Part model, mm, in its own coordinate system. A direction names the side the tool comes from. Give positions to 0.01 mm unless a question says otherwise; leave off trailing zeros. Write each loop counter-clockwise with the first axis right and the second up, starting at its lowest first coordinate (ties: lowest second). Pieces come first, ordered by that corner, then holes. Notation, with made-up numbers: M -33.5,-13.75 L -12.5,-13.75 A21 ccw -12.5,-4.75 Z; hole C 44,83.25 d2. An arc over 180 degrees is marked long. Answer as CSV lines item,"result". Start each with the question number.
1) Slice it at A-A, the plane z = 24. Give the cut face in (x, y), plus the area to 3 significant figures.
2) Tool access for faces 5 (the cylindrical face through (-3.22, -24.54, 1.43)), 6 (the cylindrical face through (0, -2, 58)): list every direction of +Z, -Z, +X, -X, +Y, -Y with a clear straight run to the whole face (end or side of a thin tool).
3) Mould opens along X. For faces 1 (the cylindrical face through (-4.336, 19.524, 1.43)), 2 (the flat face through (-1.9, -20.1, 0)), 3 (the conical face through (-2.579, -19.641, 37.395)), 4 (the flat face through (0, 0, 2.9)) say: pulls with the +X half, pulls with the -X half, needs draft (parallel to the pull), parting line crosses it, or undercut.
4) Pin check, flat tips, straight feed: pin 1 Ø3 at (y, z) = (-4.5, 25) entering from +X; pin 2 Ø8 at (y, z) = (16.5, 36.5) entering from -X; pin 3 Ø1.5 at (y, z) = (-10, 34.5) entering from -X; pin 4 Ø6 at (x, z) = (8, 53.5) entering from -Y. Stop position of each tip, or through.
5) Wall check: line 1 along Y through (x, z) = (0, 1.7); line 2 along Z through (x, y) = (3.5, -9.5); line 3 along Z through (x, y) = (16, -18.5). Give the ranges that are in metal, low to high. Write a range as from..to.
Autodesk Fusion 360 part; units mm, degrees
sketch "Skizze1" plane through (0, 0, 0) normal (0, 0, 1) x (1, 0, 0)
  circle A0 centre (0, 0) radius 24.75
  circle A1 centre (0, 0) radius 20
  dimension "d1" = 49.5
  dimension "d4" = 40
extrude "Extrusion1" add sketch "Skizze1" along normal blind 2.9
sketch "Skizze2" plane through (0, 0, 0) normal (0, 1, 0) x (1, 0, 0)
  line L0 (-24.75, -2.9) -> (24.75, -2.9)
  line L1 (-24.75, 0) -> (24.75, 0)
  line L2 (22.65, -2.9) -> (22.65, -7.9)
  line L3 (22.65, -7.9) -> (22.65, -12.9)
  line L4 (22.65, -12.9) -> (22.65, -17.9)
  line L5 (22.65, -17.9) -> (22.5, -22.8977)
  line L6 (22.5, -22.8977) -> (22, -27.8727)
  line L7 (22, -27.8727) -> (21.15, -32.7999)
  line L8 (21.15, -32.7999) -> (19.75, -37.5999)
  line L9 (19.75, -37.5999) -> (18.1, -42.3198)
  line L10 (0, -2.9) -> (0, -41.75) construction
  line L11 (18.1, -42.3198) -> (15.05, -49.9)
  line L12 (15.05, -49.9) -> (0, -49.9)
  line L13 (0, -49.9) -> (0, -2.9)
  dimension "d6" = 5
  dimension "d8" = 22.65
  dimension "d9" = 22.65
  dimension "d10" = 22.65
  dimension "d11" = 22.65
  dimension "d12" = 22.5
  dimension "d13" = 22
  dimension "d14" = 21.15
  dimension "d15" = 19.75
  dimension "d17" = 18.1
  dimension "d18" = 47
  dimension "d20" = 15.05
  dimension "d21" = 8.1708
  dimension "d22" = 7.5802
revolve "Drehen1" add sketch "Skizze2" angle 360 about axis through (0, 0, 49.9) along (0, 0, -1)
fillet "Abrundung1" radius 28 6 edges at (-16.8751, -6.5452, 42.3198) (-18.4135, -7.1419, 37.5999) (-19.7187, -7.6482, 32.7999) (-20.5112, -7.9555, 27.8727) (-20.9774, -8.1363, 22.8977) (-21.1172, -8.1906, 17.9)
fillet "Abrundung2" radius 1 1 edges at (-21.1172, 8.1906, 2.9)
sketch "Skizze3" plane through (0, 0, 49.9) normal (0, 0, 1) x (-1, 0, 0)
  circle A0 centre (0, 0) radius 15.05
  circle A1 centre (0, 0) radius 2
  dimension "d28" = 4
extrude "Extrusion2" add sketch "Skizze3" along normal blind 16 contours A1
equation "d8 = ( 45.3 / 2 ) * 1 mm"
equation "d9 = ( 45.3 / 2 ) * 1 mm"
equation "d10 = ( 45.3 / 2 ) * 1 mm"
equation "d11 = ( 45.3 / 2 ) * 1 mm"
equation "d12 = ( 45.0 / 2 ) * 1 mm"
equation "d13 = ( 44 / 2 ) * 1 mm"
equation "d14 = ( 42.3 / 2 ) * 1 mm"
equation "d15 = ( 39.5 / 2 ) * 1 mm"
equation "d17 = ( 36.2 / 2 ) * 1 mm"
equation "d20 = ( 30.1 / 2 ) * 1 mm"
Found:
1,outline,"C 0,0 d44.78"
1,area,"1,570 mm²"
2,face 5,"+Z, -Z"
2,face 6,"+Z"
3,face 1,"undercut"
3,face 2,"needs draft"
3,face 3,"parting line crosses it"
3,face 4,"undercut"
4,pin 1,"x = 22.13"
4,pin 2,"x = -16.03"
4,pin 3,"x = -18.54"
4,pin 4,"through"
5,line 1,"-24.75..-20, 20..24.75"
5,line 2,"2.9..49.9"
5,line 3,"0..2.9"
